For this review, take the finished solid that the model builds, in its own axes (mm). A direction names the side the tool comes from. Give positions to 0.01 mm unless a question says otherwise; leave off trailing zeros. Loops run counter-clockwise (first coordinate to the right, second up) from the corner with the lowest first, then second, coordinate; pieces in that order, holes last. Notation, with made-up numbers: (8.5, 25.5) - (41.5, 25.5) arc R23 ccw to (41.5, 40.5) - close; hole circle Ø6 at (59, 73). An arc over 180 degrees is marked (long way). Answer as CSV lines item,"result".
Autodesk Inventor part; units mm, degrees
ref_plane "C1_XY" through (0, 0, 0) normal (0, 0, 1) x (1, 0, 0)
ref_plane "C1_YZ" through (0, 0, 0) normal (1, 0, 0) x (0, 1, 0)
ref_plane "C1_ZX" through (0, 0, 0) normal (0, 1, 0) x (0, 0, 1)
sketch "Sketch_1" plane through (0, 0, 0) normal (0, 0, 1) x (1, 0, 0)
  line L0 (-15, 4) -> (-13, 4)
  line L1 (-13, 4) -> (-13, 8.25)
  line L2 (-13, 8.25) -> (-9.6642, 8.25)
  line L3 (-9.6642, 8.25) -> (-6, 4.5858)
  line L4 (-6, 4.5858) -> (-6, 0.5196)
  line L5 (-6, 0.5196) -> (-5.7, 0)
  line L6 (-5.7, 0) -> (-6, -0.5196)
  line L7 (-6, -0.5196) -> (-6, -4.5858)
  line L8 (-6, -4.5858) -> (-9.6642, -8.25)
  line L9 (-9.6642, -8.25) -> (-13, -8.25)
  line L10 (-13, -8.25) -> (-13, -4)
  line L11 (-13, -4) -> (-15, -4)
  line L12 (-15, -4) -> (-15, -13)
  arc A0 (-15, -13) -> (-13, -15) centre (-13, -13) ccw
  line L13 (-13, -15) -> (-4, -15)
  line L14 (-4, -15) -> (-4, -13)
  line L15 (-4, -13) -> (-8.25, -13)
  line L16 (-8.25, -13) -> (-8.25, -9.6642)
  line L17 (-8.25, -9.6642) -> (-4.5858, -6)
  line L18 (-4.5858, -6) -> (-0.5196, -6)
  line L19 (-0.5196, -6) -> (0, -5.7)
  line L20 (0, -5.7) -> (0.5196, -6)
  line L21 (0.5196, -6) -> (4.5858, -6)
  line L22 (4.5858, -6) -> (8.25, -9.6642)
  line L23 (8.25, -9.6642) -> (8.25, -13)
  line L24 (8.25, -13) -> (4, -13)
  line L25 (4, -13) -> (4, -15)
  line L26 (4, -15) -> (13, -15)
  arc A1 (13, -15) -> (15, -13) centre (13, -13) ccw
  line L27 (15, -13) -> (15, -4)
  line L28 (15, -4) -> (13, -4)
  line L29 (13, -4) -> (13, -8.25)
  line L30 (13, -8.25) -> (9.6642, -8.25)
  line L31 (9.6642, -8.25) -> (6, -4.5858)
  line L32 (6, -4.5858) -> (6, -0.5196)
  line L33 (6, -0.5196) -> (5.7, 0)
  line L34 (5.7, 0) -> (6, 0.5196)
  line L35 (6, 0.5196) -> (6, 4.5858)
  line L36 (6, 4.5858) -> (9.6642, 8.25)
  line L37 (9.6642, 8.25) -> (13, 8.25)
  line L38 (13, 8.25) -> (13, 4)
  line L39 (13, 4) -> (15, 4)
  line L40 (15, 4) -> (15, 13)
  arc A2 (15, 13) -> (13, 15) centre (13, 13) ccw
  line L41 (13, 15) -> (4, 15)
  line L42 (4, 15) -> (4, 13)
  line L43 (4, 13) -> (8.25, 13)
  line L44 (8.25, 13) -> (8.25, 9.6642)
  line L45 (8.25, 9.6642) -> (4.5858, 6)
  line L46 (4.5858, 6) -> (0.5196, 6)
  line L47 (0.5196, 6) -> (0, 5.7)
  line L48 (0, 5.7) -> (-0.5196, 6)
  line L49 (-0.5196, 6) -> (-4.5858, 6)
  line L50 (-4.5858, 6) -> (-8.25, 9.6642)
  line L51 (-8.25, 9.6642) -> (-8.25, 13)
  line L52 (-8.25, 13) -> (-4, 13)
  line L53 (-4, 13) -> (-4, 15)
  line L54 (-4, 15) -> (-13, 15)
  arc A3 (-13, 15) -> (-15, 13) centre (-13, 13) ccw
  line L55 (-15, 13) -> (-15, 4)
extrude "Extrusion1" add sketch "Sketch_1" against normal blind 30
sketch "Sketch2" plane through (0, 0, -30) normal (0, 0, -1) x (-1, 0, 0)
  point P0 (0, 0)
hole "Hole1" at (0, 0, -30) direction (0, 0, 1) diameter 6.8 depth 140
sketch "Sketch3" plane through (0, 0, -30) normal (0, 0, -1) x (-1, 0, 0)
  point P0 (-11.6, 11.6)
hole "Hole2" at (11.6, 11.6, -30) direction (0, 0, 1) diameter 4.2 depth 140
pattern_linear "Rectangular Pattern1" count 2 spacing 23.2 along (-1, 0, 0) count 2 spacing 23.2 along (0, -1, 0) of "Hole2"
ref_plane "C1_XY" through (0, 0, 0) normal (0, 0, 1) x (1, 0, 0)
ref_plane "C1_YZ" through (0, 0, 0) normal (1, 0, 0) x (0, 1, 0)
ref_plane "C1_ZX" through (0, 0, 0) normal (0, 1, 0) x (0, 0, 1)
ref_plane "to_frame_cap1_XY" through (0, 0, 0) normal (0, 0, 1) x (1, 0, 0)
ref_plane "to_frame_cap1_YZ" through (0, 0, 0) normal (1, 0, 0) x (0, 1, 0)
ref_plane "to_frame_cap1_ZX" through (0, 0, 0) normal (0, 1, 0) x (0, 0, 1)
ref_plane "to_frame_cap2_XY" through (0, 0, -140) normal (0, 0, -1) x (1, 0, 0)
ref_plane "to_frame_cap2_YZ" through (0, 0, -140) normal (1, 0, 0) x (0, -1, 0)
ref_plane "to_frame_cap2_ZX" through (0, 0, -140) normal (0, -1, 0) x (0, 0, -1)
properties part number "HFS6-3030-30"
1) Consider section B-B on x = 6.5. Write out the cut boundary in (y, z), and give its area (3 significant figures).
From the geometry:
outline,"(-15, -30) - (-13, -30) - (-13, 0) - (-15, 0) - close; (-7.91, -30) - (-5.09, -30) - (-5.09, 0) - (-7.91, 0) - close; (5.09, -30) - (7.91, -30) - (7.91, 0) - (5.09, 0) - close; (13, -30) - (15, -30) - (15, 0) - (13, 0) - close"
area,"290 mm^2"
2) Wall thickness on line 1 (X direction, y = -4.5, z = -12.5); line 2 (X direction, y = 11.6, z = -16): over which ranges is each line inside the solid? List them lowest first. Write a range as from..to.
From the geometry:
line 1,"x = -15..-13, -6..6, 13..15"
line 2,"x = -15..-13.7, -9.5..-8.25, 8.25..9.5, 13.7..15"
3) Machinability: for faces 1 (the flat face through (15, -9, -15)), 2 (the flat face through (4, -14, -15)), 3 (the flat face through (-6.392, 7.806, -14.79)), 4 (the flat face through (14, 4, -15)), 5 (the flat face through (-15, -8, -15)), which of the approach directions +Z, -Z, +X, -X, +Y, -Y give a long, thin tool a straight path to every point of the face, cutting with its end or side? Answer none if there is none.
From the geometry:
face 1,"+Z, -Z, +X, +Y, -Y"
face 2,"+Z, -Z, -Y"
face 3,"+Z, -Z"
face 4,"+Z, -Z, +X"
face 5,"+Z, -Z, -X, +Y, -Y"
4) Draft analysis for pull direction Y (two halves, no side actions). For faces 6 (the flat face through (-9, -15, -15)), 7 (the flat face through (4, 14, -15)), 8 (the flat face through (-7.806, -6.392, -14.79)), state which applies: pulls with the +Y half, pulls with the -Y half, needs draft (parallel to the pull), parting line crosses it, or undercut.
From the geometry:
face 6,"pulls with the -Y half"
face 7,"needs draft"
face 8,"undercut"
5) Consider section C-C on z = -18.5. Count the separate pieces of the cut face and the enclosed holes in it, and give its area (3 significant figures).
From the geometry:
separate pieces,"1"
enclosed holes,"5"
area,"332 mm^2"
6) Consider section A-A on y = 11.6. Write out the cut boundary in (x, z), and give its area (3 significant figures).
From the geometry:
outline,"(-15, -30) - (-13.7, -30) - (-13.7, 0) - (-15, 0) - close; (-9.5, -30) - (-8.25, -30) - (-8.25, 0) - (-9.5, 0) - close; (8.25, -30) - (9.5, -30) - (9.5, 0) - (8.25, 0) - close; (13.7, -30) - (15, -30) - (15, 0) - (13.7, 0) - close"
area,"153 mm^2"
7) Insertion check: P1, Ø4, axis at x = 5, y = -10, coming from the +Z side; P2, Ø1.5, axis at x = 1.5, z = -14, coming from the +Y side; P3, Ø2, axis at x = 2.5, z = -11, coming from the -Y side; P4, Ø2, axis at y = -2.5, z = -18, coming from the -X side. Each pin has a flat end and moves straight along its axis. Give the tip position at first contact, or say it passes through.
From the geometry:
P1,"passes through"
P2,"stops at y = 6"
P3,"stops at y = -6"
P4,"stops at x = -6"
